from build123d import *

# Parameters (mm, degrees)
SKETCH1_W           = 31
SKETCH1_H           = 43
BOSS_EXTRUDE1_DEPTH = 2
SKETCH2_W           = 5
SKETCH2_H           = 2
CUT_EXTRUDE1_DEPTH  = 2
SKETCH3_R           = 4.5
SKETCH3_W           = 5
SKETCH3_H           = 5
SKETCH3_W_2         = 2
SKETCH3_H_2         = 2
CUT_EXTRUDE2_DEPTH  = 2


with BuildPart() as part:
    # Sketch1 → Boss-Extrude1 (new body)
    with BuildSketch(Plane(origin=(0, 0, 0), x_dir=(1, 0, 0), z_dir=(0, 1, 0))):
        Rectangle(SKETCH1_W, SKETCH1_H)
    extrude(amount=BOSS_EXTRUDE1_DEPTH)

    # Sketch2 → Cut-Extrude1 (cut)
    with BuildSketch(Plane(origin=(0, 2, 0), x_dir=(1, 0, 0), z_dir=(0, 1, 0))):
        with Locations((11, 20.5)):
            Rectangle(SKETCH2_W, SKETCH2_H)
        with Locations((-11, 20.5)):
            Rectangle(SKETCH2_W, SKETCH2_H)
    extrude(amount=-CUT_EXTRUDE1_DEPTH, mode=Mode.SUBTRACT)

    # Sketch3 → Cut-Extrude2 (cut)
    with BuildSketch(Plane(origin=(0, 2, 0), x_dir=(1, 0, 0), z_dir=(0, 1, 0))):
        with Locations((0, 10.405013978)):
            Circle(SKETCH3_R)
        with Locations((11, -10)):
            Rectangle(SKETCH3_W, SKETCH3_H)
        with Locations((14.5, -17)):
            Rectangle(SKETCH3_W_2, SKETCH3_H)
        with Locations((6, -20.5)):
            Rectangle(SKETCH3_W, SKETCH3_H_2)
        with Locations((-14.5, -17)):
            Rectangle(SKETCH3_W_2, SKETCH3_H)
        with Locations((-6, -20.5)):
            Rectangle(SKETCH3_W, SKETCH3_H_2)
        with Locations((14.5, 12)):
            Rectangle(SKETCH3_W_2, SKETCH3_H)
        with Locations((-14.5, 12)):
            Rectangle(SKETCH3_W_2, SKETCH3_H)
    extrude(amount=-CUT_EXTRUDE2_DEPTH, mode=Mode.SUBTRACT)


solid = part.part
Build history of the part. All positions in model axes, mm. A direction names the side the tool comes from. Coordinates: 2 decimals unless noted, no trailing zeros. Order: outer loops, then holes, each group sorted by start corner. A loop starts at its lowest first (then second) coordinate and runs counter-clockwise, first axis right, second up. Notation, with made-up numbers: M 70,71.25 L 90,71.25 A8 ccw 90,78.25 Z; hole C -7.5,-24.75 d11. An arc over 180 degrees is marked long. One line per question, with ' | ' between items. Start each with the question number.
Q1. Probe L1, parallel to Z at x = 0, y = 1.1; L2, parallel to X at y = 0.75, z = 9; L3, parallel to Z at x = 13, y = 0.8. List the from-to ranges inside material, lowest first. Write a range as from..to.
Q2. Flat gauge pins, fed straight in: pin 1 Ø1 at (x, y) = (-11, 0.5) entering from -Z; pin 2 Ø1 at (y, z) = (0.5, -12.5) entering from +X; pin 3 Ø1.5 at (x, z) = (-8, -15.5) entering from -Y; pin 4 Ø1 at (y, z) = (0.5, 16) entering from -X. Where does each tip first touch, or does it go through?
Q3. Saw through at D-D (x = -7). List the corners of the cut face in (y, z).
Q4. 3-axis set-ups, long thin cutter, end or side, ignore diameter. For faces 1 (the face through (-8.5, 1, 21)), 2 (the face through (-13.5, 1, -20)), 3 (the face through (13.5, 1, 10)): which of +Z, -Z, +X, -X, +Y, -Y reach the whole face in a straight line?
Q5. Saw through at C-C (y = 1.05). Count the separate pieces of the cut face and the enclosed holes in it, then the cut area to 3 significant figures.
Q6. Saw through at A-A (x = 0). List the corners of the cut face in (y, z).
Q7. Saw through at B-B (x = 9). List the corners of the cut face in (y, z), then the cut area to 3 significant figures.
Q8. Two-plate mould, pull along Z, no slides. Class faces 4 (the face through (11, 1, -19.5)), 5 (the face through (8.5, 1, 10)), 6 (the face through (-3.5, 1, 21)), 7 (the face through (6, 1, 19.5)): +Z half, -Z half, draft (parallel to the pull), parting line (faces both ways), or undercut.
Check values:
1) L1: z = -21.5..-14.91, -5.91..21.5 | L2: x = -15.5..8.5, 13.5..15.5 | L3: z = -19.5..7.5, 12.5..21.5
2) pin 1: stops at z = -19.5 | pin 2: stops at x = 13.5 | pin 3: stops at y = 0 | pin 4: stops at x = -13.5
3) outline: M 0,-21.5 L 2,-21.5 L 2,19.5 L 0,19.5 Z
4) face 1: +Z, +Y, -Y | face 2: -Z, +Y, -Y | face 3: +Y, -Y
5) separate pieces: 1 | enclosed holes: 2 | area: 1,160 mm2
6) outline: M 0,-21.5 L 2,-21.5 L 2,-14.91 L 0,-14.91 Z; M 0,-5.91 L 2,-5.91 L 2,21.5 L 0,21.5 Z
7) outline: M 0,-19.5 L 2,-19.5 L 2,7.5 L 0,7.5 Z; M 0,12.5 L 2,12.5 L 2,21.5 L 0,21.5 Z | area: 72.0 mm2
8) face 4: -Z half | face 5: undercut | face 6: draft | face 7: +Z half
